Here's how the part is built. I have some questions about the finished solid (model axes, mm). Coordinates: 2 decimals unless noted, no trailing zeros. Answer as CSV lines item,"result". Start each with the question number.
Q1. For pin 1 Ø1.5 at (y, z) = (-69.5, -2) entering from -X (3 decimals); pin 2 Ø2.5 at (x, z) = (-90, -1.5) entering from -Y (3 decimals); pin 3 Ø1.5 at (y, z) = (73.5, -2) entering from +X (3 decimals), each with a flat end and sliding along its axis, tell me the tip position at first contact or that it passes through.
Q2. Thinking about a two-plate mould opening in X: for faces 1 (the face through (-203.2, -3, -14)), 2 (the face through (-1, 1, -3.048)), 3 (the face through (-103, 103, 0)), 4 (the face through (203.2, -3, -14)), which applies, released by +X, released by -X, zero draft, split by the parting line, or undercut?
Q3. I need wall thicknesses on line 1 (X direction, y = 14.5, z = -1.5) (3 decimals). Which ranges of the line are inside material? Lowest first, please.
from build123d import *

# Parameters (mm, degrees)
F0_W     = 406.4
F0_H     = 406.4
F1_DEPTH = 25.4
F2_W     = 425.3633022308
F2_H     = 428.5580217838
F2_W_2   = 196.85
F2_H_2   = 196.85
F3_DEPTH = 3.048


# Not quite as in the source:
# - a feature names something its author has since deleted; it is built from what else it names


with BuildPart() as f1:
    # F0 (on Top) → F1 (new body)
    with BuildSketch(Plane.XY):
        Rectangle(F0_W, F0_H)
    extrude(amount=-F1_DEPTH)

    # F2 (on Top) → F3 (cut)
    with BuildSketch(Plane.XY):
        Rectangle(F2_W, F2_H)
        with Locations((-101.6, -101.6)):
            Rectangle(F2_W_2, F2_H_2, mode=Mode.SUBTRACT)
        with Locations((101.6, -101.6)):
            Rectangle(F2_W_2, F2_H_2, mode=Mode.SUBTRACT)
        with Locations((-101.6, 101.6)):
            Rectangle(F2_W_2, F2_H_2, mode=Mode.SUBTRACT)
        with Locations((101.6, 101.6)):
            Rectangle(F2_W_2, F2_H_2, mode=Mode.SUBTRACT)
    extrude(amount=-F3_DEPTH, mode=Mode.SUBTRACT)


solid = f1.part
Here are the results:
1,pin 1,"stops at x = -200.025"
1,pin 2,"stops at y = -200.025"
1,pin 3,"stops at x = 200.025"
2,face 1,"released by -X"
2,face 2,"undercut"
2,face 3,"zero draft"
2,face 4,"released by +X"
3,line 1,"x = -200.025 to -3.175, 3.175 to 200.025"
